Geometry: final body of the model. Coordinates: model frame, mm. Face numbers are marked on the shaded views. Coordinates: 2 decimals unless noted, no trailing zeros. Order: outer loops, then holes, each group sorted by start corner. A loop starts at its lowest first (then second) coordinate and runs counter-clockwise, first axis right, second up. Notation, with made-up numbers: M 12,80.25 L 43,80.25 A23 ccw 43,97.25 Z; hole C 4.25,-24.75 d5. An arc over 180 degrees is marked long. One line per question, with ' | ' between items.
Autodesk Inventor part; units mm, degrees
ref_plane "YZ Plane" through (0, 0, 0) normal (1, 0, 0) x (0, 1, 0)
ref_plane "XZ Plane" through (0, 0, 0) normal (0, 1, 0) x (-1, 0, 0)
ref_plane "XY Plane" through (0, 0, 0) normal (0, 0, 1) x (1, 0, 0)
sketch "Sketch1" plane through (0, 0, 0) normal (0, 0, 1) x (1, 0, 0)
  line L0 (-55, -55) -> (55, -55)
  line L1 (55, -55) -> (55, 55)
  line L2 (55, 55) -> (-55, 55)
  line L3 (-55, 55) -> (-55, -55)
  line L4 (-55, -55) -> (55, 55) construction
  line L5 (55, -55) -> (-55, 55) construction
  point P0 (0, 0)
  dimension "d0" = 110
  dimension "d1" = 110
extrude "Extrusion1" add sketch "Sketch1" along normal blind 5
sketch "Sketch2" plane through (0, 0, 5) normal (0, 0, 1) x (1, 0, 0)
  point P0 (0, 0)
  point P1 (-49, 49)
  point P2 (49, 49)
  point P3 (-49, -49)
  point P4 (49, -49)
  dimension "d11" = 98
  dimension "d12" = 98
  dimension "d13" = 49
  dimension "d14" = 49
hole "Hole1" at (-49, 49, 5) at (49, 49, 5) at (-49, -49, 5) at (49, -49, 5) direction (0, 0, -1) diameter 4.5 depth 8.8 tip angle 118
fillet "Fillet1" radius 4 4 edges at (55, 55, 2.5) (55, -55, 2.5) (-55, -55, 2.5) (-55, 55, 2.5)
sketch "Sketch3" plane through (0, 0, 5) normal (0, 0, 1) x (1, 0, 0)
  line L0 (-6.1969, -19) -> (-19, -19)
  line L1 (-19, -19) -> (-19, 19)
  line L2 (-19, 19) -> (19, 19)
  line L3 (19, 19) -> (-6.1969, -19)
  line L4 (-6.1969, -19) -> (-19, 19) construction
  line L5 (-19, -19) -> (19, 19) construction
  line L6 (-55, 51) -> (-55, -51)
  arc A0 (-12.2164, 19) -> (-12.2164, -19) centre (11, 0) ccw
  arc A1 (-19, -12.2164) -> (19, -12.2164) centre (0, 11) ccw
  arc A2 (12.2164, -19) -> (12.2164, 19) centre (-11, 0) ccw
  arc A3 (19, 12.2164) -> (-19, 12.2164) centre (0, -11) ccw
  line L7 (-19, -7) -> (-19, 7)
  line L8 (-91.8281, -7) -> (-18.1719, -7)
  line L9 (-18.1719, -7) -> (-18.1719, 7)
  line L10 (-18.1719, 7) -> (-91.8281, 7)
  line L11 (-91.8281, 7) -> (-91.8281, -7)
  line L12 (-91.8281, -7) -> (-18.1719, 7) construction
  line L13 (-18.1719, -7) -> (-91.8281, 7) construction
  point P0 (0, 0)
  point P1 (0, 0)
  point P2 (-19, 0)
  point P3 (0, -19)
  point P4 (19, 0)
  point P5 (0, 19)
  point P6 (-15.2369, 15.7631)
  point P7 (-14.9878, 14.9878)
  point P8 (-46.7631, -15.7631)
  point P9 (14.9878, -14.9878)
  point P10 (-14.9878, -14.9878)
  point P11 (14.9878, 14.9878)
  point P12 (-55, 0)
  point P13 (-55, 7)
  point P14 (-55, -7)
  point P15 (-18.1719, -7)
  dimension "d18" = 38
  dimension "d19" = 38
  dimension "d20" = 30
  dimension "d23" = 360
  dimension "d28" = 42.3919
  dimension "d30" = 14
extrude "Extrusion2" cut sketch "Sketch3" against normal blind 3 contours A1 A0 L9 A3 A2 L3 | L3 A2 A1 | L8 L1 A0 | A0 L9 | L8 L6 L10 L1 | L1 L10 A0
fillet "Fillet2" radius 3 4 edges at (14.9878, -14.9878, 3.5) (-14.9878, 14.9878, 3.5) (-18.1719, -7, 3.5) (-18.1719, 7, 3.5)
sketch "Sketch4" plane through (0, 0, 5) normal (0, 0, 1) x (1, 0, 0)
  line L0 (55, -51) -> (55, 51) construction
  line L1 (50, 20) -> (50, 0) construction
  point P0 (0, 0)
  point P1 (55, 0)
  point P2 (50, 10)
  dimension "d40" = 20
  dimension "d43" = 10
  dimension "d44" = 5
hole "Hole2" at (50, 20, 5) at (50, 0, 5) direction (0, 0, -1) diameter 4.5 depth 14.2 tip angle 118
fillet "Fillet3" radius 2 2 edges at (-55, -7, 3.5) (-55, 7, 3.5)
equation "\"d0\" = pcb_size"
equation "\"d1\" = pcb_size"
properties part number "support_camera"
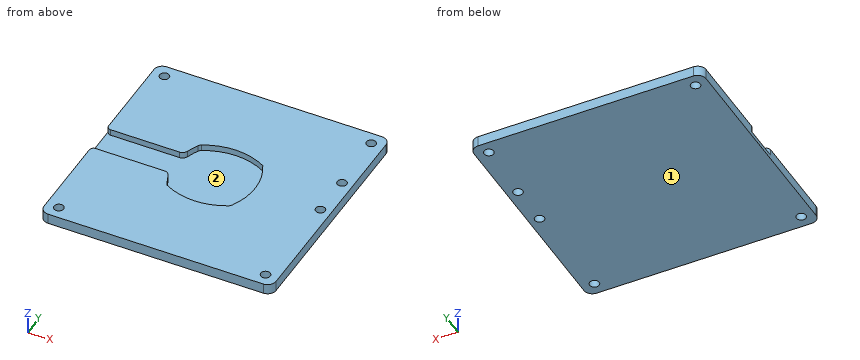
1. Section D-D, the plane x = 10.5. Output: boundary loops of the cut face in (y, z).
Response values:
outline: M -55,0 L 55,0 L 55,5 L 17.1,5 L 17.1,2 L -17.1,2 L -17.1,5 L -55,5 Z
2. Section C-C, the plane y = 0. Output: boundary loops of the cut face in (x, z).
Response values:
outline: M -55,0 L 47.75,0 L 47.75,5 L 19,5 L 19,2 L -55,2 Z; M 52.25,0 L 55,0 L 55,5 L 52.25,5 Z
3. Section A-A, the plane x = -49. Output: boundary loops of the cut face in (y, z), and give its area (3 significant figures).
Response values:
outline: M -55,0 L -51.25,0 L -51.25,5 L -55,5 Z; M -46.75,0 L 46.75,0 L 46.75,5 L 7,5 L 7,2 L -7,2 L -7,5 L -46.75,5 Z; M 51.25,0 L 55,0 L 55,5 L 51.25,5 Z | area: 463 mm^2
4. Section B-B, the plane y = -49. Output: boundary loops of the cut face in (x, z).
Response values:
outline: M -55,0 L -51.25,0 L -51.25,5 L -55,5 Z; M -46.75,0 L 46.75,0 L 46.75,5 L -46.75,5 Z; M 51.25,0 L 55,0 L 55,5 L 51.25,5 Z
5. Draft query along Y for the marked faces 1 and 2. Return one class per face: pulls with the +Y half, pulls with the -Y half, needs draft (parallel to the pull), parting line crosses it, or undercut.
Response values:
face 1: needs draft | face 2: undercut
6. Pin query (flat end, axial travel): P1, Ø4, axis at x = 49, y = 49, coming from the -Z side; P2, Ø5, axis at x = 49, y = -49, coming from the +Z side. Return the tip coordinate at first contact, or that it passes through.
Response values:
P1: passes through | P2: stops at z = 5
7. Material intervals for line 1 (Y direction, x = -49, z = 2.4); line 2 (Y direction, x = -49, z = 1.7), sorted ascending. Write a range as [from, to].
Response values:
line 1: y = [-55, -51.25], [-46.75, -7], [7, 46.75], [51.25, 55] | line 2: y = [-55, -51.25], [-46.75, 46.75], [51.25, 55]
